```python
from build123d import *

# Parameters (mm, degrees)
BOSS_EXTRUDE1_DEPTH = 17.5
CUT_EXTRUDE1_DEPTH  = 1
HOLE1_D             = 4.4
HOLE2_D             = 4.4
HOLE3_D             = 8.4
HOLE4_D             = 8.4
FILLET1_R           = 10


with BuildPart() as part:
    # Sketch1 → Boss-Extrude1 (new body)
    with BuildSketch(Plane.XY.offset(17.5)):
        with BuildLine():
            Line((8.706689755, -31.721063073), (-3.596567561, 15.283592096))
            Line((-3.596567561, 15.283592096), (-25.765781543, 25.213668746))
            ThreePointArc((-25.765781543, 25.213668746), (-36.126401787, 23.029680686), (-37.239092363, 12.5))
            Line((-37.239092363, 12.5), (-7.794228634, -38.5))
            ThreePointArc((-7.794228634, -38.5), (3.420035495, -42.324863795), (8.706689755, -31.721063073))
        make_face()
    extrude(amount=-BOSS_EXTRUDE1_DEPTH)

    # Sketch2 → Cut-Extrude1 (cut)
    with BuildSketch(Plane(origin=(-22.516660498, -13, 0), x_dir=(0, 0, 1), z_dir=(-0.866025403784438, -0.500000000000001, 0))):
        with BuildLine():
            Line((9.791987556, 18.365854028), (10.909334809, 19.444863729))
            Line((10.909334809, 19.444863729), (9.791987556, 20.523873429))
            ThreePointArc((9.791987556, 20.523873429), (7.25, 19.444863729), (9.791987556, 18.365854028))
        make_face()
    extrude(amount=-CUT_EXTRUDE1_DEPTH, mode=Mode.SUBTRACT)

    # Hole1 (through all)
    with Locations(Plane(origin=(0, 0, 0), x_dir=(-1, 0, 0), z_dir=(0, 0, -1))):
        with Locations((12.057368355, 8.116025404)):
            Hole(HOLE1_D / 2)

    # Hole2 (through all)
    with Locations(Plane(origin=(0, 0, 0), x_dir=(-1, 0, 0), z_dir=(0, 0, -1))):
        with Locations((12.124355653, -13)):
            Hole(HOLE2_D / 2)

    # Hole3 (through all)
    with Locations(Plane(origin=(0, 0, 0), x_dir=(-1, 0, 0), z_dir=(0, 0, -1))):
        with Locations((0, -34)):
            Hole(HOLE3_D / 2)

    # Hole4 (through all)
    with Locations(Plane(origin=(0, 0, 0), x_dir=(-1, 0, 0), z_dir=(0, 0, -1))):
        with Locations((29.444863729, 17)):
            Hole(HOLE4_D / 2)

    # Fillet1
    fillet1_edges = [part.edges().sort_by_distance(p)[0] for p in [
        (-3.596567561, 15.283592096, 8.75),
    ]]
    fillet(fillet1_edges, radius=FILLET1_R)


solid = part.part
```
Input: part model. Units: mm. Frame: model coordinates. A direction names the side the tool comes from. Round coordinates to 2 decimals unless told otherwise and drop trailing zeros. Order: outer loops, then holes, each group sorted by start corner. A loop starts at its lowest first (then second) coordinate and runs counter-clockwise, first axis right, second up. Notation, with made-up numbers: (44.5, -11) - (82.5, -11) arc R26 ccw to (82.5, 7) - close; hole circle Ø5 at (-3.75, 23.5). An arc over 180 degrees is marked (long way). One line per question, with ' | ' between items. Start each with the question number.
1) Contact query for flat-ended pins moving along their axis: P1, Ø2, axis at y = -7.5, z = 11.5, coming from the +X side; P2, Ø8, axis at x = -19.5, z = 6, coming from the -Y side; P3, Ø7, axis at x = -12.06, y = 8.12, coming from the +Z side; P4, Ø10, axis at y = -30, z = 15, coming from the -X side. Output: stop coordinate, or through.
2) Cut plane C-C, the plane z = 8. Return the cut outline in (x, y), then the cut area to 3 significant figures.
3) Cut plane D-D, the plane z = 3. Return the cut outline in (x, y).
4) Set-up query: faces 1 (the flat face through (-32.078, 4.547, 10.358)), 2 (the cylindrical face through (-4.387, 14.532, 8.628)). Return all of +Z, -Z, +X, -X, +Y, -Y with unobstructed straight access to the full face (end or side cutting, diameter ignored); none if empty.
5) Cut plane B-B, the plane x = 0. Return the cut outline in (y, z).
6) Cut plane A-A, the plane y = -13. Return the cut outline in (x, z), then the cut area to 3 significant figures.
7) Ray query, probe 1 along X at (y, z) = (-11.5, 1.5) (3 decimals); probe 2 along X at (y, z) = (18, 10.75); probe 3 along Y at (x, z) = (-30, 11.25). Return the intervals inside material, ascending.
8) Pull-direction query (Z, two-part tool) for faces 3 (the flat face through (-15, -8, 0)), 4 (the flat face through (-31.54, 3.61, 10.34)), 5 (the cylindrical face through (3.252, -42.392, 8.872)); classes: +Z half, -Z half, draft (parallel to the pull), parting line (faces both ways), or undercut.
Worked out:
1) P1: stops at x = 2.63 | P2: stops at y = -25.15 | P3: stops at z = 17.5 | P4: stops at x = -15.59
2) outline: (-37.24, 12.5) - (-32.89, 4.96) - (-32.02, 5.46) - (-30.72, 3.21) - (-31.59, 2.71) - (-7.79, -38.5) arc R9 ccw to (8.71, -31.72) - (-2.38, 10.65) arc R10 ccw to (-7.97, 17.24) - (-25.77, 25.21) arc R9 ccw to start; hole circle Ø8.4 at (-29.44, 17); hole circle Ø4.4 at (-12.12, -13); hole circle Ø4.4 at (-12.06, 8.12); hole circle Ø8.4 at (0, -34) | area: 1,560 mm^2
3) outline: (-37.24, 12.5) - (-7.79, -38.5) arc R9 ccw to (8.71, -31.72) - (-2.38, 10.65) arc R10 ccw to (-7.97, 17.24) - (-25.77, 25.21) arc R9 ccw to start; hole circle Ø8.4 at (-29.44, 17); hole circle Ø4.4 at (-12.12, -13); hole circle Ø4.4 at (-12.06, 8.12); hole circle Ø8.4 at (0, -34)
4) face 1: none | face 2: +Z, -Z, +X, +Y
5) outline: (-43, 0) - (-38.2, 0) - (-38.2, 17.5) - (-43, 17.5) - close; (-29.8, 0) - (1.54, 0) - (1.54, 17.5) - (-29.8, 17.5) - close
6) outline: (-22.52, 0) - (-14.32, 0) - (-14.32, 17.5) - (-22.52, 17.5) - close; (-9.92, 0) - (3.81, 0) - (3.81, 17.5) - (-9.92, 17.5) - close | area: 384 mm^2
7) probe 1: x = -23.383 to -13.734, -10.515 to 3.414 | probe 2: x = -38.39 to -33.52, -25.37 to -9.66 | probe 3: y = -0.04 to 12.84, 21.16 to 25.98
8) face 3: -Z half | face 4: undercut | face 5: draft
